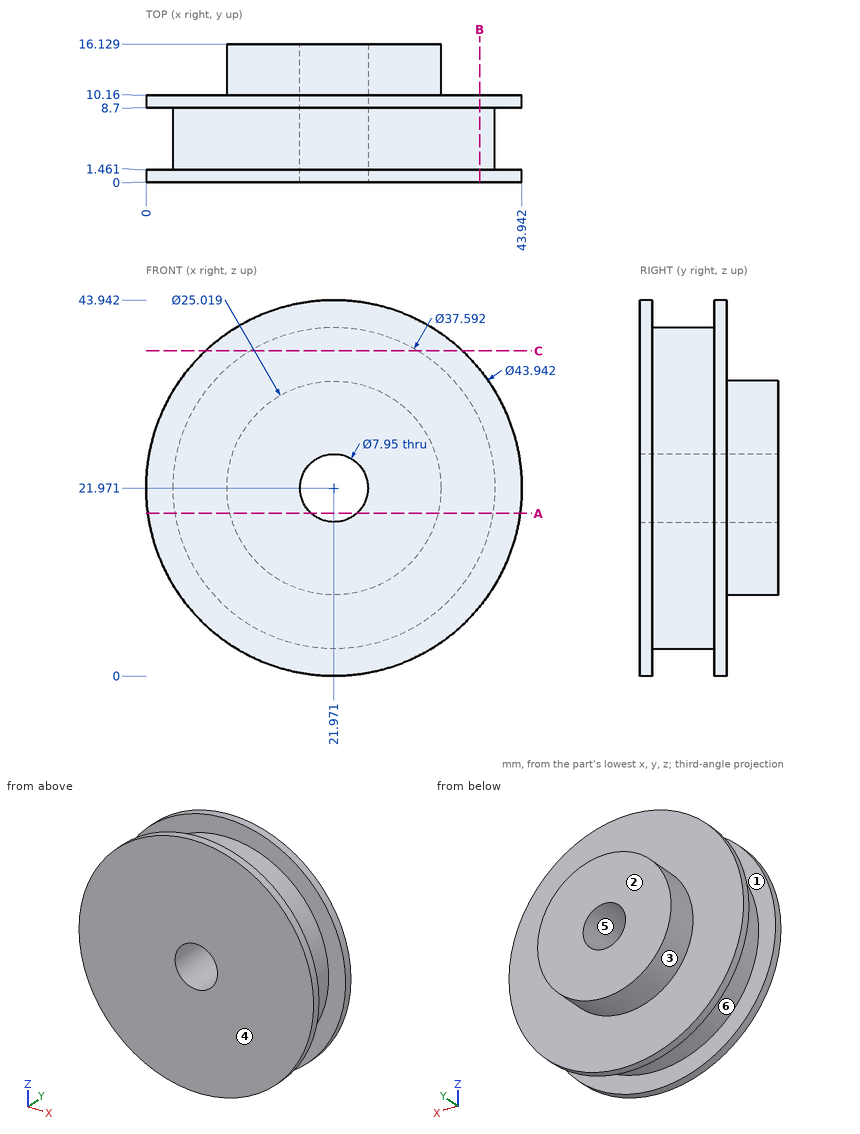
Study the drawing (mm; zero at the part's minimum x, y, z) and answer. A direction names the side the tool comes from. Give positions to 0.01 mm unless a question says otherwise; leave off trailing zeros. Order: outer loops, then holes, each group sorted by start corner. A loop starts at its lowest first (then second) coordinate and runs counter-clockwise, first axis right, second up. Notation, with made-up numbers: (16, -35) - (62, -35) arc R16 ccw to (62, -24) - close; hole circle Ø11 at (-22, 22.5). An arc over 180 degrees is marked (long way). Answer in a Markdown table with one row per item. Add a question column.
Q1. Find the intervals of material crossed by line 1 along Y through (x, z) = (42.5, 16.5); line 2 along Y through (x, z) = (30, 6); line 3 along Z through (x, y) = (32, 8.5) (1 decimal), in increasing order. Write a range as [from, to].
Q2. Given P1, Ø1, axis at x = 8.5, y = 10.5, coming from the +Z side (1 decimal); P2, Ø6, axis at y = 2, z = 25, coming from the -X side; P3, Ø2, axis at x = 21, y = 4, coming from the +Z side; P4, Ø5, axis at y = 5, z = 21.5, coming from the +X side, each flat-ended and moving along its own axis, determine where each tip first touches the part or whether it passes through.
Q3. The part is cut by section C-C (z = 38). Determine the outline of the cut face in (x, y) (1 decimal).
Q4. Which of the six approach directions +Z, -Z, +X, -X, +Y, -Y give full straight-line access (tool end or side, diameter ignored) to the marked faces 1, 2 and 3?
Q5. The part is cut by section A-A (z = 19). Determine the outline of the cut face in (x, y), then the cut area to 3 significant figures.
Q6. The part is cut by section B-B (x = 39). Determine the outline of the cut face in (y, z) (1 decimal), then the cut area to 3 significant figures.
Q7. For a pull along Z with two mould halves and no side action, classify the marked faces 4, 5 and 6 as released by +Z, released by -Z, zero draft, split by the parting line, or undercut.
Determined:
| question | item | result |
|---|---|---|
| 1 | line 1 | y = [0, 1.46], [8.7, 10.16] |
| 1 | line 2 | y = [0, 10.16] |
| 1 | line 3 | z = [6.1, 37.9] |
| 2 | P1 | stops at z = 39.6 |
| 2 | P2 | stops at x = 0 |
| 2 | P3 | stops at z = 40.77 |
| 2 | P4 | stops at x = 40.77 |
| 3 | outline | (6.9, 0) - (37, 0) - (37, 1.5) - (31.8, 1.5) - (31.8, 8.7) - (37, 8.7) - (37, 10.2) - (6.9, 10.2) - (6.9, 8.7) - (12.2, 8.7) - (12.2, 1.5) - (6.9, 1.5) - close |
| 4 | face 1 | none |
| 4 | face 2 | +Z, -Z, +X, -X, +Y |
| 4 | face 3 | +Y |
| 5 | outline | (0.2, 0) - (19.33, 0) - (19.33, 16.13) - (9.82, 16.13) - (9.82, 10.16) - (0.2, 10.16) - (0.2, 8.7) - (3.41, 8.7) - (3.41, 1.46) - (0.2, 1.46) - close; (24.61, 0) - (43.74, 0) - (43.74, 1.46) - (40.53, 1.46) - (40.53, 8.7) - (43.74, 8.7) - (43.74, 10.16) - (34.12, 10.16) - (34.12, 16.13) - (24.61, 16.13) - close |
| 5 | area | 456 mm² |
| 6 | outline | (0, 8.1) - (1.5, 8.1) - (1.5, 14) - (8.7, 14) - (8.7, 8.1) - (10.2, 8.1) - (10.2, 35.9) - (8.7, 35.9) - (8.7, 29.9) - (1.5, 29.9) - (1.5, 35.9) - (0, 35.9) - close |
| 6 | area | 196 mm² |
| 7 | face 4 | zero draft |
| 7 | face 5 | undercut |
| 7 | face 6 | split by the parting line |
